```python
from build123d import *

# Parameters (mm, degrees)
BOSS_EXTRUDE1_DEPTH     = 2.5399999999999996
BOSS_EXTRUDE3_DEPTH     = 12.7
BOSS_EXTRUDE6_DEPTH     = 2.54
BOSS_EXTRUDE7_DEPTH     = 25.4
BOSS_EXTRUDE8_START     = 10.16
BOSS_EXTRUDE8_DEPTH     = 15.239999999999998
FILLET1_R               = 2.5399999999999996
FILLET2_ANGLE           = 169.351542
FILLET3_R               = 0.762
CUT_EXTRUDE1_DEPTH      = 93.8296161634462
CUT_EXTRUDE1_DEPTH_BACK = 93.8296161634462
SKETCH3_R               = 1.9050000000000038
SKETCH3_R_2             = 1.9049999999999983


with BuildPart() as part:
    # Sketch2 → Boss-Extrude1 (new body)
    with BuildSketch(Plane.XY):
        with BuildLine():
            Line((0, 85.598), (0, 0))
            Line((0, 0), (14.804819963776673, 1e-17))
            ThreePointArc((14.804819963776595, -3.0553e-13), (2.268412192290537, 24.14357981267628), (21.081999999999496, 43.793589476431805))
            Line((21.082000000000004, 43.79358947643172), (21.082, 85.598))
            Line((21.082, 85.598), (0, 85.598))
        make_face()
    extrude(amount=BOSS_EXTRUDE1_DEPTH)



with BuildPart() as body_2:
    # Sketch2<4> → Boss-Extrude3 (new body)
    with BuildSketch(Plane.XY):
        with BuildLine():
            ThreePointArc((21.082000000000008, 41.98179341867554), (3.82144132339004, 21.53078406363614), (19.714710561456986, 2.0606e-13))
            Line((19.714710561456965, 2e-17), (25.399999983196594, 2e-17))
            ThreePointArc((25.399999983196587, -3.55e-15), (4.685437224641706, 18.657176878292418), (21.082000000000004, 41.20348674265231))
            Line((21.082000000000004, 41.20348674265231), (21.082000000000004, 41.98179341867554))
        make_face()
        with BuildLine():
            ThreePointArc((25.400000000000105, 42.418000000000006), (23.230011510307612, 42.30867154338064), (21.082000000000008, 41.98179341867554))
            Line((21.082000000000004, 41.98179341867554), (21.082000000000004, 41.20348674265231))
            ThreePointArc((21.082000000000004, 41.20348674265231), (23.229176869936293, 41.542562774482604), (25.39999999999965, 41.656000000000006))
            Line((25.400000000000002, 41.656000000000006), (25.400000000000002, 42.418000000000006))
        make_face()
        with BuildLine():
            Line((25.399999983196594, 2e-17), (19.714710561456965, 2e-17))
            ThreePointArc((19.714710561456986, 2.0606e-13), (22.531936193178055, -0.5706520603518008), (25.4000000000001, -0.7620000000000076))
            Line((25.40000000000001, -0.7620000000000147), (25.40000000000001, 0))
        make_face()
    extrude(amount=BOSS_EXTRUDE3_DEPTH)


with BuildPart() as part_1:
    add(part.part)

    add(body_2.part)  # Boss-Extrude6 merges body 2
    # Sketch2<9> → Boss-Extrude6 (add)
    with BuildSketch(Plane.XY):
        with BuildLine():
            ThreePointArc((21.081999999999496, 43.793589476431805), (2.268412192290537, 24.14357981267628), (14.804819963776595, -3.0553e-13))
            Line((14.804819963776673, 1e-17), (19.714710561456965, 2e-17))
            ThreePointArc((19.714710561456986, 2.0606e-13), (3.82144132339004, 21.53078406363614), (21.082000000000008, 41.98179341867554))
            Line((21.082000000000004, 41.98179341867554), (21.082000000000004, 43.79358947643172))
        make_face()
    extrude(amount=BOSS_EXTRUDE6_DEPTH)

    # Sketch2<10> → Boss-Extrude7 (add)
    with BuildSketch(Plane.XY):
        with BuildLine():
            Line((25.4, 85.598), (21.082, 85.598))
            Line((21.082, 85.598), (21.082000000000004, 43.79358947643172))
            ThreePointArc((21.081999999999496, 43.793589476431805), (23.231644734511608, 44.095179877299884), (25.39999999999975, 44.196))
            Line((25.400000000000002, 44.196), (25.4, 85.598))
        make_face()
        with BuildLine():
            ThreePointArc((25.39999999999975, 44.196), (23.231644734511608, 44.095179877299884), (21.081999999999496, 43.793589476431805))
            Line((21.082000000000004, 43.79358947643172), (21.082000000000004, 41.98179341867554))
            ThreePointArc((21.082000000000008, 41.98179341867554), (23.230011510307612, 42.30867154338064), (25.400000000000105, 42.418000000000006))
            Line((25.400000000000002, 42.418000000000006), (25.400000000000002, 44.196))
        make_face()
    extrude(amount=BOSS_EXTRUDE7_DEPTH)

    # Sketch2<12> → Boss-Extrude8 (add)
    with BuildSketch(Plane.XY.offset(BOSS_EXTRUDE8_START)):
        with BuildLine():
            Line((19.714710561456965, 2e-17), (14.804819963776673, 1e-17))
            ThreePointArc((14.804819963776595, -3.0553e-13), (19.952306910260432, -1.8961295542866416), (25.400000000000006, -2.539999999999999))
            Line((25.40000000000001, -2.5400000000000063), (25.40000000000001, -0.7620000000000147))
            ThreePointArc((25.4000000000001, -0.7620000000000076), (22.531936193178055, -0.5706520603518008), (19.714710561456986, 2.0606e-13))
        make_face()
        with BuildLine():
            ThreePointArc((21.081999999999496, 43.793589476431805), (2.268412192290537, 24.14357981267628), (14.804819963776595, -3.0553e-13))
            Line((14.804819963776673, 1e-17), (19.714710561456965, 2e-17))
            ThreePointArc((19.714710561456986, 2.0606e-13), (3.82144132339004, 21.53078406363614), (21.082000000000008, 41.98179341867554))
            Line((21.082000000000004, 41.98179341867554), (21.082000000000004, 43.79358947643172))
        make_face()
    extrude(amount=BOSS_EXTRUDE8_DEPTH)

    # Fillet1
    fillet1_edges = [part_1.edges().sort_by_distance(p)[0] for p in [
        (21.082, 63.78989670933777, 2.5399999999999996),
        (3.8214413233900366, 21.530784063636144, 2.54),
    ]]
    fillet(fillet1_edges, radius=FILLET1_R)

    # Fillet2: read off the stored shape, not the designer's step
    # Fillet2 outline → Fillet2 (revolve)
    with BuildSketch(Plane(origin=(25.4, 20.828, 0), x_dir=(-0.1847826086956513, 0.982779419566583, 0), z_dir=(0.982779419566583, 0.1847826086956513, 0))):
        with BuildLine():
            ThreePointArc((21.59, 7.736994428), (22.082186532, 9.239678693), (23.368, 10.16))
            Line((23.368, 10.16), (21.59, 10.16))
            Line((21.59, 10.16), (21.59, 7.736994428))
        make_face()
    revolve(axis=Axis((25.4, 20.828, 0), (0, 0, 1)), revolution_arc=FILLET2_ANGLE)

    # Fillet3
    fillet3_edges = [part_1.edges().sort_by_distance(p)[0] for p in [
        (3.809999999999814, 20.827999999999818, 12.7),
    ]]
    fillet(fillet3_edges, radius=FILLET3_R - 0.0001)  # a hair under: the kernel refuses the full size

    # Sketch3 → Cut-Extrude1 (cut, two sides: drawn at the far end of the back side and taken through both)
    with BuildSketch(Plane(origin=(0, 0, 0), x_dir=(0, 0, -1), z_dir=(1, 0, 0)).offset(-CUT_EXTRUDE1_DEPTH_BACK)):
        with Locations(Location((-15.24, 76.2, 0), (0, 0, 90))):
            Circle(SKETCH3_R)
        with Locations(Location((-15.239999999999998, 49.53, 0), (0, 0, 90))):
            Circle(SKETCH3_R_2)
    extrude(amount=CUT_EXTRUDE1_DEPTH + CUT_EXTRUDE1_DEPTH_BACK, mode=Mode.SUBTRACT)


solid = part_1.part
```
The model under review builds one solid part; all positions refer to its coordinate system, in mm. A direction names the side the tool comes from. Give positions to 0.01 mm unless a question says otherwise; leave off trailing zeros. Write each loop counter-clockwise with the first axis right and the second up, starting at its lowest first coordinate (ties: lowest second). Pieces come first, ordered by that corner, then holes. Notation, with made-up numbers: M 70,12 L 90,12 A24 ccw 90,23 Z; hole C -31,28 d8. An arc over 180 degrees is marked long. Write item = value, one per line. Start each with the question number.
Q1. Machinability: for faces 4 (the face through (3.815, 20.353, 19.347)), 5 (the face through (5.57, 12.29, 5.53)), 6 (the face through (22, 85.598, 9)), 7 (the face through (10, 0, 1)), 8 (the face through (2.093, 19.141, 17.673)), which of the approach directions +Z, -Z, +X, -X, +Y, -Y give a long, thin tool a straight path to every point of the face, cutting with its end or side? Answer none if there is none.
Q2. Clearance check with flat-ended pins moving along their axes: pin 1 (1.5 mm diameter, centred on x = 10, z = 2, fed in from -Y); pin 2 (4 mm diameter, centred on y = 74.5, z = 22, fed in from -X); pin 3 (5 mm diameter, centred on x = 5, z = 10.5, fed in from +Y); pin 4 (3 mm diameter, centred on y = 49.53, z = 15.24, fed in from -X). State where each tip first meets the part, or that it passes through.
Q3. Mouldability with a two-part tool opening along Z and no side actions: class faces 1 (the face through (4.577, 20.37, 6.261)), 2 (the face through (23.21, 48.02, 14.08)), 3 (the face through (7, 53, 2.54)) as released by +Z, released by -Z, zero draft, split by the parting line, or undercut.
Q4. We need section C-C (y = 58.5). State the section outline as (x, z) points.
Q5. We need section B-B (y = 76.2). State the section outline as (x, z) points (3 decimals), plus the area to 3 significant figures.
Q6. For line 1 (Z direction, x = 23.55, y = 76.2) (3 decimals); line 2 (Y direction, x = 22, z = 15.24) (3 decimals); line 3 (Y direction, x = 24.3, z = 15.24) (3 decimals), list the stretches that pass through material, from the lowest coordinate up.
Q7. We need section D-D (z = 20). State the section outline as (x, y) points.
Q8. We need section A-A (z = 15.24). State the section outline as (x, y) points (3 decimals).
Result set:
q1.face_4 = +Z, +X
q1.face_5 = -X
q1.face_6 = +Z, -Z, +X, -X, +Y
q1.face_7 = -Z, -X, -Y
q1.face_8 = +Z, -X
q2.pin_1 = 0
q2.pin_2 = 21.08
q2.pin_3 = 35.85
q2.pin_4 = through
q3.face_1 = zero draft
q3.face_2 = undercut
q3.face_3 = released by +Z
q4.outline = M 0,0 L 25.4,0 L 25.4,25.4 L 21.08,25.4 L 21.08,5.08 A2.54 cw 18.54,2.54 L 0,2.54 Z
q5.outline = M 0,0 L 25.4,0 L 25.4,13.335 L 21.082,13.335 L 21.082,5.08 A2.54 cw 18.542,2.54 L 0,2.54 Z; M 21.082,17.145 L 25.4,17.145 L 25.4,25.4 L 21.082,25.4 Z
q5.area = 148 mm2
q6.line_1 = 0 to 13.335, 17.145 to 25.4
q6.line_2 = -2.291 to -0.493, 42.149 to 47.625, 51.435 to 74.295, 78.105 to 85.598
q6.line_3 = -2.514 to -0.734, 42.39 to 47.625, 51.435 to 74.295, 78.105 to 85.598
q7.outline = M 21.08,43.79 A23.37 ccw 25.4,-2.54 L 25.4,-0.76 A21.59 cw 25.4,42.42 L 25.4,85.6 L 21.08,85.6 Z
q8.outline = M 21.082,43.794 A23.368 ccw 25.4,-2.54 L 25.4,-0.762 A21.59 cw 25.4,42.418 L 25.4,47.625 L 21.082,47.625 Z; M 21.082,51.435 L 25.4,51.435 L 25.4,74.295 L 21.082,74.295 Z; M 21.082,78.105 L 25.4,78.105 L 25.4,85.598 L 21.082,85.598 Z
